```python
from build123d import *

# Parameters (mm, degrees)
SKETCH1_R           = 32.75
BOSS_EXTRUDE1_DEPTH = 12.3
SKETCH2_R           = 7
BOSS_EXTRUDE2_DEPTH = 7.1
SKETCH4_R           = 25
CUT_EXTRUDE1_DEPTH  = 3


with BuildPart() as part:
    # Sketch1 → Boss-Extrude1 (new body)
    with BuildSketch(Plane(origin=(0, 0, 0), x_dir=(1, 0, 0), z_dir=(0, 1, 0))):
        with Locations(Location((0, 0, 0), (0, 0, 270))):
            Circle(SKETCH1_R)
    extrude(amount=BOSS_EXTRUDE1_DEPTH)

    # Sketch2 → Boss-Extrude2 (add)
    with BuildSketch(Plane(origin=(0, 12.3, 0), x_dir=(1, 0, 0), z_dir=(0, 1, 0))):
        with Locations(Location((0, 0, 0), (0, 0, 270))):
            Circle(SKETCH2_R)
    extrude(amount=BOSS_EXTRUDE2_DEPTH)

    # Sketch4 → Cut-Extrude1 (cut)
    with BuildSketch(Plane.XZ):
        with Locations(Location((0, 0, 0), (0, 0, 270))):
            Circle(SKETCH4_R)
    extrude(amount=-CUT_EXTRUDE1_DEPTH, mode=Mode.SUBTRACT)


solid = part.part
```
The model under review builds one solid part; all positions refer to its coordinate system, in mm. A direction names the side the tool comes from. Round coordinates to 2 decimals unless told otherwise and drop trailing zeros. Write each loop counter-clockwise with the first axis right and the second up, starting at its lowest first coordinate (ties: lowest second). Pieces come first, ordered by that corner, then holes.
(1) We need section C-C on y = 16.5. Give the boundary of the cut face in (x, z).
(2) Machinability: for faces 1 (the cylindrical face through (-6.834, 15.8, -1.517)), 2 (the cylindrical face through (7.509, 1.479, -23.846)), 3 (the flat face through (-24.1, 0, -7.4)), which of the approach directions +Z, -Z, +X, -X, +Y, -Y give a long, thin tool a straight path to every point of the face, cutting with its end or side? Answer none if there is none.
(3) Mouldability with a two-part tool opening along Z and no side actions: class faces 4 (the flat face through (8, 12.3, 0)), 5 (the flat face through (0, 3, 0)), 6 (the cylindrical face through (9.837, 6.064, 31.238)) as +Z half, -Z half, draft (parallel to the pull), parting line (faces both ways), or undercut.
(4) We need section B-B on x = 0. Give the boundary of the cut face in (y, z).
(5) We need section D-D on x = -17.5. Give the boundary of the cut face in (y, z), and give its area (3 significant figures).
(6) Insertion check: pin 1 (6 mm diameter, centred on x = 11.5, z = 22, fed in from +Y); pin 2 (3 mm diameter, centred on x = -6.5, y = 12.5, fed in from +Z); pin 3 (5 mm diameter, centred on y = 3.5, z = -16.5, fed in from +X). Each pin has a flat end and moves straight along its axis. Give the tip position at first contact, or say it passes through.
(7) We need section A-A on z = 0. Give the boundary of the cut face in (x, y).
(8) Wall thickness on L1, parallel to X at y = 1.5, z = 0; L2, parallel to Y at x = -6, z = -27; L3, parallel to Y at x = 23.5, z = -2: over which ranges is each line inside the solid? List them lowest first.
Findings below:
1. outline: circle Ø14 at (0, 0)
2. face 1: +Y
2. face 2: -Y
2. face 3: +Z, -Z, +X, -X, -Y
3. face 4: draft
3. face 5: undercut
3. face 6: parting line
4. outline: (0, -32.75) - (12.3, -32.75) - (12.3, -7) - (19.4, -7) - (19.4, 7) - (12.3, 7) - (12.3, 32.75) - (0, 32.75) - (0, 25) - (3, 25) - (3, -25) - (0, -25) - close
5. outline: (0, -27.68) - (12.3, -27.68) - (12.3, 27.68) - (0, 27.68) - (0, 17.85) - (3, 17.85) - (3, -17.85) - (0, -17.85) - close
5. area: 574 mm2
6. pin 1: stops at y = 12.3
6. pin 2: stops at z = 32.36
6. pin 3: stops at x = 29.61
7. outline: (-32.75, 0) - (-25, 0) - (-25, 3) - (25, 3) - (25, 0) - (32.75, 0) - (32.75, 12.3) - (7, 12.3) - (7, 19.4) - (-7, 19.4) - (-7, 12.3) - (-32.75, 12.3) - close
8. L1: x = -32.75 to -25, 25 to 32.75
8. L2: y = 0 to 12.3
8. L3: y = 3 to 12.3
